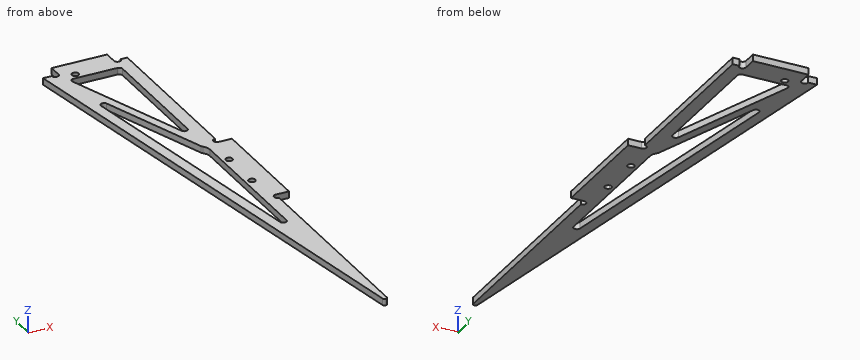
from build123d import *

# Parameters (mm, degrees)
EXTRUDE_1_DEPTH     = 3
SKETCH_2_R          = 1.525
CUT_EXTRUDE_1_DEPTH = 40
SKETCH_4_W          = 25
SKETCH_4_H          = 6
SKETCH_4_W_2        = 6
SKETCH_4_H_2        = 50
EXTRUDE_2_DEPTH     = 3
SKETCH_5_R          = 1.525
CUT_EXTRUDE_2_DEPTH = 40
CUT_EXTRUDE_3_DEPTH = 60
FILLET_1_R          = 1
FILLET_2_R          = 1.5
EXTRUDE_3_DEPTH     = 3
FILLET_3_R          = 5
FILLET_4_R          = 1.5


with BuildPart() as part:
    # 草图1 → 凸台-拉伸1 (new body)
    with BuildSketch(Plane.XY):
        Polygon((-38, 0), (0, 0), (0, -240), align=None)
    extrude(amount=EXTRUDE_1_DEPTH)

    # 草图2 → 切除-拉伸1 (cut)
    with BuildSketch(Plane.XY.offset(3)):
        with Locations((-3, -115)):
            Circle(SKETCH_2_R)
        with Locations((-3, -95)):
            Circle(SKETCH_2_R)
        with Locations((-25, -3)):
            Circle(SKETCH_2_R)
    extrude(amount=-CUT_EXTRUDE_1_DEPTH, mode=Mode.SUBTRACT)

    # 草图4 → 凸台-拉伸2 (add)
    with BuildSketch(Plane.XY.offset(3)):
        with Locations((-18.5, 3)):
            Rectangle(SKETCH_4_W, SKETCH_4_H)
        with Locations((3, -105)):
            Rectangle(SKETCH_4_W_2, SKETCH_4_H_2)
    extrude(amount=-EXTRUDE_2_DEPTH)

    # 草图5 → 切除-拉伸2 (cut)
    with BuildSketch(Plane(origin=(0, 0, 0), x_dir=(-1, 0, 0), z_dir=(0, 0, -1))):
        with Locations((0, -78.475)):
            Circle(SKETCH_5_R)
        with Locations((0, -131.525)):
            Circle(SKETCH_5_R)
        with Locations((4.475, 0)):
            Circle(SKETCH_5_R)
        with Locations((32.525, 0)):
            Circle(SKETCH_5_R)
    extrude(amount=-CUT_EXTRUDE_2_DEPTH, mode=Mode.SUBTRACT)

    # 草图6 → 切除-拉伸3 (cut)
    with BuildSketch(Plane(origin=(0, 0, 0), x_dir=(-1, 0, 0), z_dir=(0, 0, -1))):
        Polygon((6, -6), (6, -170.132932669), (31.987714339, -6), align=None)
    extrude(amount=-CUT_EXTRUDE_3_DEPTH, mode=Mode.SUBTRACT)

    # 圆角1
    fillet_1_edges = [part.edges().sort_by_distance(p)[0] for p in [
        (0, -240, 1.5),
    ]]
    fillet(fillet_1_edges, radius=FILLET_1_R)

    # 圆角2
    fillet_2_edges = [part.edges().sort_by_distance(p)[0] for p in [
        (-6, -6, 1.5),
        (-31.987714339, -6, 1.5),
        (-6, -170.132932669, 1.5),
    ]]
    fillet(fillet_2_edges, radius=FILLET_2_R)

    # 草图7 → 凸台-拉伸3 (add)
    with BuildSketch(Plane(origin=(0, 0, 0), x_dir=(-1, 0, 0), z_dir=(0, 0, -1))):
        with BuildLine():
            Line((7.888469575, -79.942320526), (33.26058288, -7.184345364))
            ThreePointArc((33.26058288, -7.184345364), (32.030659174, -4.637329919), (29.483643729, -5.867253624))
            Line((29.483643729, -5.867253624), (4.111530425, -78.625228786))
            ThreePointArc((4.111530425, -78.625228786), (5.34145413, -81.172244231), (7.888469575, -79.942320526))
        make_face()
    extrude(amount=-EXTRUDE_3_DEPTH)

    # 圆角3
    fillet_3_edges = [part.edges().sort_by_distance(p)[0] for p in [
        (-6, -81.283774656, 1.5),
    ]]
    fillet(fillet_3_edges, radius=FILLET_3_R)

    # 圆角4
    fillet_4_edges = [part.edges().sort_by_distance(p)[0] for p in [
        (-6, -73.209786217, 1.5),
        (-30.585668879, -14.855023959, 1.5),
        (-29.4373525, -6, 1.5),
    ]]
    fillet(fillet_4_edges, radius=FILLET_4_R)


solid = part.part
Geometry: final body of the model. Coordinates: model frame, mm. Round coordinates to 2 decimals unless told otherwise and drop trailing zeros. Loops run counter-clockwise (first coordinate to the right, second up) from the corner with the lowest first, then second, coordinate; pieces in that order, holes last. Notation, with made-up numbers: M 17,38 L 48,38 A22 ccw 48,75 Z; hole C -6,-35 d7. An arc over 180 degrees is marked long. Put each result on its own line as item: value. Start each with the question number.
(1) Section query B-B (z = 1.05). State how many separate pieces and enclosed holes the cut face has, then the cut area to 3 significant figures.
(2) Section query C-C (x = 2.5). Return loops of the section in (y, z), then the cut area to 3 significant figures.
(3) Section query A-A (y = -144.5). Return loops of the section in (x, z).
(4) Material intervals for line 1 along X through (y, z) = (-95, 1.8) (3 decimals); line 2 along Y through (x, z) = (3.5, 1.8); line 3 along X through (y, z) = (-115, 0.95) (3 decimals), sorted ascending. Write a range as [from, to].
(5) Contact query for flat-ended pins moving along their axis: pin 1 Ø0.9 at (y, z) = (-31.5, 1.5) entering from +X; pin 2 Ø2.5 at (x, y) = (-3, -95) entering from -Z; pin 3 Ø0.9 at (y, z) = (4, 2) entering from +X; pin 4 Ø1.5 at (x, z) = (2, 2) entering from +Y. Output: stop coordinate, or through.
(6) Section query D-D (y = -46.5). Return loops of the section in (x, z), then the cut area to 3 significant figures.
Findings below:
1. separate pieces: 1
1. enclosed holes: 5
1. area: 3,190 mm2
2. outline: M -130,0 L -80,0 L -80,3 L -130,3 Z
2. area: 150 mm2
3. outline: M -15.12,0 L -10.06,0 L -10.06,3 L -15.12,3 Z; M -6,0 L 0,0 L 0,3 L -6,3 Z
4. line 1: x = [-22.958, -17.896], [-6, -4.525], [-1.475, 6]
4. line 2: y = [-130, -80]
4. line 3: x = [-19.792, -14.729], [-6, -4.525], [-1.475, 6]
5. pin 1: stops at x = 0
5. pin 2: passes through
5. pin 3: stops at x = -6
5. pin 4: stops at y = -80
6. outline: M -30.64,0 L -25.58,0 L -25.58,3 L -30.64,3 Z; M -19.55,0 L -15.31,0 L -15.31,3 L -19.55,3 Z; M -6,0 L 0,0 L 0,3 L -6,3 Z
6. area: 45.9 mm2
